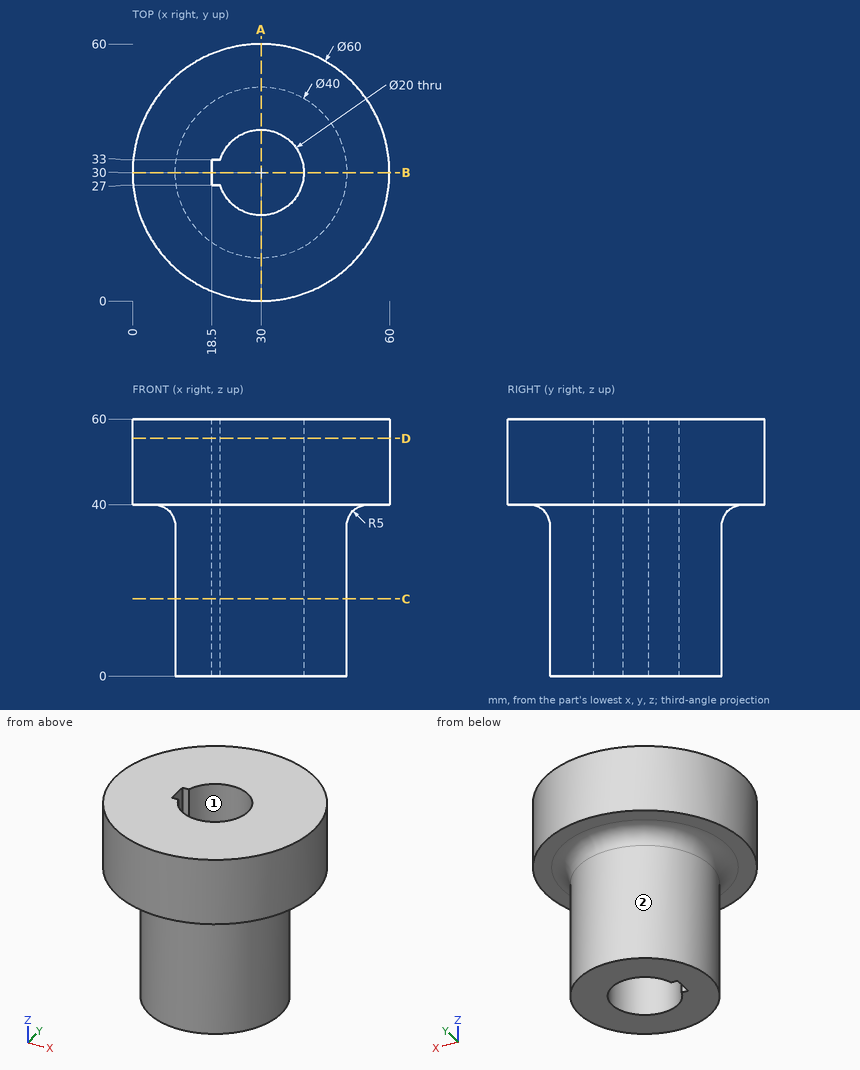
Part print with two shaded views. Sizes in mm from the minimum x, y, z corner. A direction names the side the tool comes from. Round coordinates to 2 decimals unless told otherwise and drop trailing zeros. Loops run counter-clockwise (first coordinate to the right, second up) from the corner with the lowest first, then second, coordinate; pieces in that order, holes last.
Item 1: Pin check, flat tips, straight feed: P1, Ø1.8, axis at y = 29.5, z = 32, coming from the +X side; P2, Ø1.6, axis at x = 19.5, z = 18.5, coming from the +Y side; P3, Ø1.5, axis at y = 49, z = 12.5, coming from the +X side. Stop position of each tip, or through.
Item 2: Saw through at D-D (z = 55.5). List the corners of the cut face in (x, y), then the cut area to 3 significant figures.
Item 3: Saw through at B-B (y = 30). List the corners of the cut face in (x, z), then the cut area to 3 significant figures.
Item 4: Saw through at C-C (z = 18). List the corners of the cut face in (x, y), then the cut area to 3 significant figures.
Item 5: Drill centre lines: line 1 along Y through (x, z) = (30, 31.5); line 2 along Z through (x, y) = (46, 49); line 3 along X through (y, z) = (21, 35.5). Where is each one in solid material? Low to high.
Item 6: Saw through at A-A (x = 30). List the corners of the cut face in (y, z).
Item 7: Which spindle directions (+Z, -Z, +X, -X, +Y, -Y) get a long thin tool onto all of the face, cutting with end or side? Do the marked faces 1 and 2. Say none if no direction does.
Worked answers:
1. P1: stops at x = 50
1. P2: stops at y = 47.49
1. P3: stops at x = 38.18
2. outline: circle Ø60 at (30, 30); hole (18.5, 27) - (20.46, 27) arc R10 ccw (long way) to (20.46, 33) - (18.5, 33) - close
2. area: 2,500 mm2
3. outline: (0, 40) - (5, 40) arc R5 cw to (10, 35) - (10, 0) - (18.5, 0) - (18.5, 60) - (0, 60) - close; (40, 0) - (50, 0) - (50, 35) arc R5 cw to (55, 40) - (60, 40) - (60, 60) - (40, 60) - close
3. area: 1,520 mm2
4. outline: circle Ø40 at (30, 30); hole (18.5, 27) - (20.46, 27) arc R10 ccw (long way) to (20.46, 33) - (18.5, 33) - close
4. area: 933 mm2
5. line 1: y = 10 to 20, 40 to 50
5. line 2: z = 40 to 60
5. line 3: x = 12.11 to 25.64, 34.36 to 47.89
6. outline: (0, 40) - (5, 40) arc R5 cw to (10, 35) - (10, 0) - (20, 0) - (20, 60) - (0, 60) - close; (40, 0) - (50, 0) - (50, 35) arc R5 cw to (55, 40) - (60, 40) - (60, 60) - (40, 60) - close
7. face 1: +Z, -Z
7. face 2: -Z
